from build123d import *

# Parameters (mm, degrees)
F0_W     = 190
F0_H     = 106
F1_DEPTH = 0.8
F2_W     = 190
F2_H     = 106
F2_W_2   = 36.8
F2_H_2   = 25.3
F2_W_3   = 37.2
F2_H_3   = 25.7
F2_W_4   = 188.4
F3_DEPTH = 44
F4_R     = 12.5
F5_DEPTH = 0.8


# Not quite as in the source:
# - a feature names something its author has since deleted; it is built from what else it names


with BuildPart() as f1:
    # F0 (on Top) → F1 (new body)
    with BuildSketch(Plane.XY):
        with Locations((-95, 53)):
            Rectangle(F0_W, F0_H)
    extrude(amount=F1_DEPTH)

    # F2 (on face) → F3 (join)
    with BuildSketch(Plane.XY.offset(0.8)):
        with Locations((-95, 53)):
            Rectangle(F2_W, F2_H)
        with Locations((-170.8, 13.45)):
            Rectangle(F2_W_2, F2_H_2, mode=Mode.SUBTRACT)
        with Locations((-133, 13.45)):
            Rectangle(F2_W_3, F2_H_2, mode=Mode.SUBTRACT)
        with Locations((-170.8, 39.75)):
            Rectangle(F2_W_2, F2_H_3, mode=Mode.SUBTRACT)
        with Locations((-133, 39.75)):
            Rectangle(F2_W_3, F2_H_3, mode=Mode.SUBTRACT)
        with Locations((-95, 13.45)):
            Rectangle(F2_W_3, F2_H_2, mode=Mode.SUBTRACT)
        with Locations((-57, 13.45)):
            Rectangle(F2_W_3, F2_H_2, mode=Mode.SUBTRACT)
        with Locations((-19.2, 13.45)):
            Rectangle(F2_W_2, F2_H_2, mode=Mode.SUBTRACT)
        with Locations((-95, 39.75)):
            Rectangle(F2_W_3, F2_H_3, mode=Mode.SUBTRACT)
        with Locations((-57, 39.75)):
            Rectangle(F2_W_3, F2_H_3, mode=Mode.SUBTRACT)
        with Locations((-19.2, 39.75)):
            Rectangle(F2_W_2, F2_H_3, mode=Mode.SUBTRACT)
        with Locations((-170.8, 66.25)):
            Rectangle(F2_W_2, F2_H_3, mode=Mode.SUBTRACT)
        with Locations((-133, 66.25)):
            Rectangle(F2_W_3, F2_H_3, mode=Mode.SUBTRACT)
        with Locations((-95, 66.25)):
            Rectangle(F2_W_3, F2_H_3, mode=Mode.SUBTRACT)
        with Locations((-57, 66.25)):
            Rectangle(F2_W_3, F2_H_3, mode=Mode.SUBTRACT)
        with Locations((-19.2, 66.25)):
            Rectangle(F2_W_2, F2_H_3, mode=Mode.SUBTRACT)
        with Locations((-95, 92.55)):
            Rectangle(F2_W_4, F2_H_2, mode=Mode.SUBTRACT)
    extrude(amount=F3_DEPTH)

    # F4 (on face) → F5 (join)
    with BuildSketch(Plane(origin=(0, 0, 0), x_dir=(1, 0, 0), z_dir=(0, 0, -1))):
        Circle(F4_R)
        with Locations((-190, 0)):
            Circle(F4_R)
        with Locations((-190, -106)):
            Circle(F4_R)
        with Locations((0, -106)):
            Circle(F4_R)
    extrude(amount=-F5_DEPTH)


solid = f1.part
Could you check a few things on this model? Use its own coordinates, in mm. A direction names the side the tool comes from. Coordinates: 2 decimals unless noted, no trailing zeros. Write each loop counter-clockwise with the first axis right and the second up, starting at its lowest first coordinate (ties: lowest second). Pieces come first, ordered by that corner, then holes. Notation, with made-up numbers: (7, -36.75) - (20, -36.75) arc R19 cw to (20, -26.75) - close; hole circle Ø1 at (26, 47.5). An arc over 180 degrees is marked (long way). Put each result on its own line as item: value. Start each with the question number.
Q1. I want a section at A-A on y = 110. Write out the boundary of the cut face in (x, z).
Q2. I'm going to push flat-ended pins straight in: P1, Ø2, axis at x = -26.5, y = 93, coming from the +Z side; P2, Ø20, axis at x = -4.5, y = 102.5, coming from the +Z side; P3, Ø1.5, axis at y = 44.5, z = 27, coming from the +X side; P4, Ø5, axis at x = -101, z = 10, coming from the +Y side. Where does each tip first touch, or does it pass through?
Q3. I want a section at D-D on z = 26. Count the separate pieces of the cut face and the enclosed holes in it, plus the area to 3 significant figures.
Q4. Which directions (+Z, -Z, +X, -X, +Y, -Y) give clear straight access to the entire face, cutting with the end or side of a thin tool? Please do faces 1 (the flat face through (-189.2, 40, 22)), 2 (the cylindrical face through (9.13, -8.54, 0.39)).
Q5. Thinking about a two-plate mould opening in X: for faces 3 (the flat face through (-190, 52, 22)), 4 (the flat face through (-19, 79.1, 22)), 5 (the flat face through (-193, 109, 0.8)), which applies, pulls with the +X half, pulls with the -X half, needs draft (parallel to the pull), parting line crosses it, or undercut?
Q6. Please list where these lines run through material, in increasing order: L1, parallel to Y at x = -6, z = 18; L2, parallel to X at y = 55.5, z = 39.5; L3, parallel to X at y = 101.5, z = 10.5.
Q7. I want a section at B-B on x = -7.5. Write out the boundary of the cut face in (y, z), plus the area to 3 significant figures.
Q8. I want a section at C-C on y = 77. Write out the boundary of the cut face in (x, z), plus the area to 3 significant figures.
Checks:
1. outline: (-201.84, 0) - (-178.16, 0) - (-178.16, 0.8) - (-201.84, 0.8) - close; (-11.84, 0) - (11.84, 0) - (11.84, 0.8) - (-11.84, 0.8) - close
2. P1: z = 0.8
2. P2: z = 44.8
2. P3: x = 0
2. P4: y = 106
3. separate pieces: 1
3. enclosed holes: 16
3. area: 1,170 mm²
4. face 1: +Z
4. face 2: +Z, -Z
5. face 3: pulls with the -X half
5. face 4: undercut
5. face 5: needs draft
6. L1: 0 to 0.8, 26.1 to 26.9, 52.6 to 53.4, 79.1 to 79.9, 105.2 to 106
6. L2: -190 to -189.2, -152.4 to -151.6, -114.4 to -113.6, -76.4 to -75.6, -38.4 to -37.6, -0.8 to 0
6. L3: -190 to -189.2, -0.8 to 0
7. outline: (-10, 0) - (116, 0) - (116, 0.8) - (106, 0.8) - (106, 44.8) - (105.2, 44.8) - (105.2, 0.8) - (79.9, 0.8) - (79.9, 44.8) - (79.1, 44.8) - (79.1, 0.8) - (53.4, 0.8) - (53.4, 44.8) - (52.6, 44.8) - (52.6, 0.8) - (26.9, 0.8) - (26.9, 44.8) - (26.1, 44.8) - (26.1, 0.8) - (0.8, 0.8) - (0.8, 44.8) - (0, 44.8) - (0, 0.8) - (-10, 0.8) - close
7. area: 277 mm²
8. outline: (-190, 0) - (0, 0) - (0, 44.8) - (-0.8, 44.8) - (-0.8, 0.8) - (-37.6, 0.8) - (-37.6, 44.8) - (-38.4, 44.8) - (-38.4, 0.8) - (-75.6, 0.8) - (-75.6, 44.8) - (-76.4, 44.8) - (-76.4, 0.8) - (-113.6, 0.8) - (-113.6, 44.8) - (-114.4, 44.8) - (-114.4, 0.8) - (-151.6, 0.8) - (-151.6, 44.8) - (-152.4, 44.8) - (-152.4, 0.8) - (-189.2, 0.8) - (-189.2, 44.8) - (-190, 44.8) - close
8. area: 363 mm²
